from build123d import *

# Parameters (mm, degrees)
F0_W     = 47.24663
F0_H     = 33.02
F2_DEPTH = 12.7
F1_R     = 23.687869
F3_DEPTH = 12.7
F4_R     = 13.83799
F5_DEPTH = 12.701
F6_W     = 23.371061
F6_H     = 4.762498
F8_DEPTH = 33.02
F7_W     = 24.04602
F7_H     = 4.372004
F9_DEPTH = 25.4


with BuildPart() as f2:
    # F0 (on Top) → F2 (new body)
    with BuildSketch(Plane.XY):
        with Locations((23.623315, 16.51)):
            Rectangle(F0_W, F0_H)
    extrude(amount=F2_DEPTH)

    # F1 (on Top) → F3 (join)
    with BuildSketch(Plane.XY):
        with Locations((23.615431, 1.851092)):
            Circle(F1_R)
    extrude(amount=F3_DEPTH)

    # F4 (on Top) → F5 (cut, through all)
    with BuildSketch(Plane.XY):
        with Locations((23.24864, 0)):
            Circle(F4_R)
    extrude(amount=F5_DEPTH, mode=Mode.SUBTRACT)

    # F6 (on Top) → F8 (join)
    with BuildSketch(Plane.XY):
        with Locations((11.68553, 35.401249)):
            Rectangle(F6_W, F6_H)
    extrude(amount=F8_DEPTH)

    # F7 (on Top) → F9 (join)
    with BuildSketch(Plane.XY):
        with Locations((35.279802, 35.49272)):
            Rectangle(F7_W, F7_H)
    extrude(amount=F9_DEPTH)


solid = f2.part
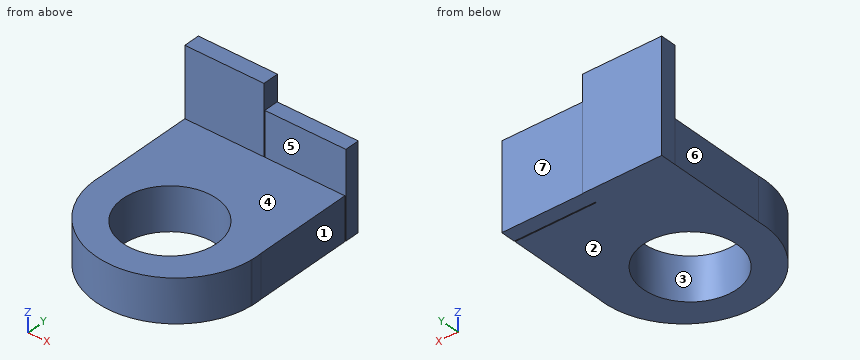
Here's how the part is built. I have some questions about the finished solid (model axes, mm). Face numbers are marked on the shaded views. A direction names the side the tool comes from. Coordinates: 2 decimals unless noted, no trailing zeros. Loops run counter-clockwise (first coordinate to the right, second up) from the corner with the lowest first, then second, coordinate; pieces in that order, holes last. Notation, with made-up numbers: (19, 36.5) -> (73, 36.5) arc R27 ccw to (73, 65.5) -> close; hole circle Ø1 at (59, -10). An arc over 180 degrees is marked (long way). Use one line per item in the form item = value. Start each with the question number.
(1) Will these pins go through, and if not, where does the flat tip stop? pin 1 (5 mm diameter, centred on x = 33, z = 20, fed in from -Y); pin 2 (18.5 mm diameter, centred on x = 6.5, z = 13, fed in from -Y); pin 3 (19 mm diameter, centred on x = 33.5, z = 7, fed in from -Y).
(2) If we section it at C-C (x = 42): Please give me the cut outline in (y, z), then the cut area to 3 significant figures.
(3) On a 3-axis mill with a long thin cutter (end or side, diameter ignored), from which of +Z, -Z, +X, -X, +Y, -Y can I reach the whole of each face in a straight line? I mean the marked faces 4, 5, 6 and 7. Say none if no direction works.
(4) If we section it at B-B (y = 5): Please give me the cut outline in (x, z), then the cut area to 3 significant figures.
(5) Please list where these lines run through material, in increasing order: line 1 along X through (y, z) = (0, 10.25); line 2 along Y through (x, z) = (26, 6.5); line 3 along Z through (x, y) = (7.5, 20.5).
(6) We'd pull the mould along X, two halves only. Please class the marked faces 1, 2 and 3: pulls with the +X half, pulls with the -X half, needs draft (parallel to the pull), parting line crosses it, or undercut.
(7) If we section it at D-D (z = 16.5): Please give me the cut outline in (x, y).
Verdict:
q1.pin_1 = 33.31
q1.pin_2 = -20.49
q1.pin_3 = -21.83
q2.outline = (-13.09, 0) -> (33.02, 0) -> (33.02, 12.7) -> (-13.09, 12.7) -> close; (33.31, 0) -> (37.68, 0) -> (37.68, 25.4) -> (33.31, 25.4) -> close
q2.area = 697 mm²
q3.face_4 = +Z, +X, -X, -Y
q3.face_5 = +Z, -Z, +X
q3.face_6 = +Z, -Z, -X, +Y
q3.face_7 = +Z, -Z, +X, +Y
q4.outline = (0, 0) -> (10.35, 0) -> (10.35, 12.7) -> (0, 12.7) -> close; (36.15, 0) -> (47.25, 0) -> (47.25, 12.7) -> (36.15, 12.7) -> close
q4.area = 272 mm²
q5.line_1 = 0 to 9.41, 37.09 to 47.23
q5.line_2 = -21.72 to -13.56, 13.56 to 33.02, 33.31 to 37.68
q5.line_3 = 0 to 12.7
q6.face_1 = pulls with the +X half
q6.face_2 = needs draft
q6.face_3 = undercut
q7.outline = (0, 33.02) -> (23.37, 33.02) -> (23.37, 33.31) -> (47.3, 33.31) -> (47.3, 37.68) -> (23.37, 37.68) -> (23.37, 37.78) -> (0, 37.78) -> close
